CAD build for the part. Positions are in the model's coordinates, mm. A direction names the side the tool comes from. Coordinates: 2 decimals unless noted, no trailing zeros. Write item = value, one per line.
Autodesk Inventor part; units mm, degrees
ref_plane "C1_XY" through (0, 0, 0) normal (0, 0, 1) x (1, 0, 0)
ref_plane "C1_YZ" through (0, 0, 0) normal (1, 0, 0) x (0, 1, 0)
ref_plane "C1_ZX" through (0, 0, 0) normal (0, 1, 0) x (0, 0, 1)
sketch "Sketch_63" plane through (0, 0, 0) normal (0, 0, 1) x (1, 0, 0)
  line L0 (-10, -7) -> (-8, -7)
  line L1 (-8, -7) -> (-8, -4)
  line L2 (-8, -4) -> (-7.0607, -4)
  line L3 (-7.0607, -4) -> (-4, -7.0607)
  line L4 (-4, -7.0607) -> (-4, -9.4804)
  line L5 (-4, -9.4804) -> (-3.7, -10)
  line L6 (-3.7, -10) -> (-4, -10.5196)
  line L7 (-4, -10.5196) -> (-4, -12.9393)
  line L8 (-4, -12.9393) -> (-7.0607, -16)
  line L9 (-7.0607, -16) -> (-8, -16)
  line L10 (-8, -16) -> (-8, -13)
  line L11 (-8, -13) -> (-10, -13)
  line L12 (-10, -13) -> (-10, -19)
  arc A0 (-10, -19) -> (-9, -20) centre (-9, -19) ccw
  line L13 (-9, -20) -> (-3, -20)
  line L14 (-3, -20) -> (-3, -18)
  line L15 (-3, -18) -> (-6, -18)
  line L16 (-6, -18) -> (-6, -17.0607)
  line L17 (-6, -17.0607) -> (-2.9393, -14)
  line L18 (-2.9393, -14) -> (-0.5196, -14)
  line L19 (-0.5196, -14) -> (0, -13.7)
  line L20 (0, -13.7) -> (0.5196, -14)
  line L21 (0.5196, -14) -> (2.9393, -14)
  line L22 (2.9393, -14) -> (6, -17.0607)
  line L23 (6, -17.0607) -> (6, -18)
  line L24 (6, -18) -> (3, -18)
  line L25 (3, -18) -> (3, -20)
  line L26 (3, -20) -> (9, -20)
  arc A1 (9, -20) -> (10, -19) centre (9, -19) ccw
  line L27 (10, -19) -> (10, 19)
  arc A2 (10, 19) -> (9, 20) centre (9, 19) ccw
  line L28 (9, 20) -> (3, 20)
  line L29 (3, 20) -> (3, 18)
  line L30 (3, 18) -> (6, 18)
  line L31 (6, 18) -> (6, 17.0607)
  line L32 (6, 17.0607) -> (2.9393, 14)
  line L33 (2.9393, 14) -> (0.5196, 14)
  line L34 (0.5196, 14) -> (0, 13.7)
  line L35 (0, 13.7) -> (-0.5196, 14)
  line L36 (-0.5196, 14) -> (-2.9393, 14)
  line L37 (-2.9393, 14) -> (-6, 17.0607)
  line L38 (-6, 17.0607) -> (-6, 18)
  line L39 (-6, 18) -> (-3, 18)
  line L40 (-3, 18) -> (-3, 20)
  line L41 (-3, 20) -> (-9, 20)
  arc A3 (-9, 20) -> (-10, 19) centre (-9, 19) ccw
  line L42 (-10, 19) -> (-10, 13)
  line L43 (-10, 13) -> (-8, 13)
  line L44 (-8, 13) -> (-8, 16)
  line L45 (-8, 16) -> (-7.0607, 16)
  line L46 (-7.0607, 16) -> (-4, 12.9393)
  line L47 (-4, 12.9393) -> (-4, 10.5196)
  line L48 (-4, 10.5196) -> (-3.7, 10)
  line L49 (-3.7, 10) -> (-4, 9.4804)
  line L50 (-4, 9.4804) -> (-4, 7.0607)
  line L51 (-4, 7.0607) -> (-7.0607, 4)
  line L52 (-7.0607, 4) -> (-8, 4)
  line L53 (-8, 4) -> (-8, 7)
  line L54 (-8, 7) -> (-10, 7)
  line L55 (-10, 7) -> (-10, -7)
  line L56 (4, 12.9393) -> (4, 8.5)
  arc A4 (4, 8.5) -> (5, 7.5) centre (5, 8.5) ccw
  line L57 (5, 7.5) -> (7, 7.5)
  arc A5 (7, 7.5) -> (8, 8.5) centre (7, 8.5) ccw
  line L58 (8, 8.5) -> (8, 16)
  line L59 (8, 16) -> (7.0607, 16)
  line L60 (7.0607, 16) -> (4, 12.9393)
  line L61 (4, -12.9393) -> (7.0607, -16)
  line L62 (7.0607, -16) -> (8, -16)
  line L63 (8, -16) -> (8, -8.5)
  arc A6 (8, -8.5) -> (7, -7.5) centre (7, -8.5) ccw
  line L64 (7, -7.5) -> (5, -7.5)
  arc A7 (5, -7.5) -> (4, -8.5) centre (5, -8.5) ccw
  line L65 (4, -8.5) -> (4, -12.9393)
  line L66 (-8, 1.7) -> (-8, -1.7)
  arc A8 (-8, -1.7) -> (-7.7, -2) centre (-7.7, -1.7) ccw
  line L67 (-7.7, -2) -> (-7.0636, -2)
  arc A9 (-6.8515, -2.0879) -> (-7.0636, -2) centre (-7.0636, -2.3) ccw
  line L68 (-6.8515, -2.0879) -> (-2.9393, -6)
  line L69 (-2.9393, -6) -> (7, -6)
  arc A10 (7, -6) -> (8, -5) centre (7, -5) ccw
  line L70 (8, -5) -> (8, 5)
  arc A11 (8, 5) -> (7, 6) centre (7, 5) ccw
  line L71 (7, 6) -> (-2.9393, 6)
  line L72 (-2.9393, 6) -> (-6.8515, 2.0879)
  arc A12 (-7.0636, 2) -> (-6.8515, 2.0879) centre (-7.0636, 2.3) ccw
  line L73 (-7.0636, 2) -> (-7.7, 2)
  arc A13 (-7.7, 2) -> (-8, 1.7) centre (-7.7, 1.7) ccw
extrude "Extrusion1" add sketch "Sketch_63" against normal blind 393
sketch "Sketch2" plane through (0, 0, -393) normal (0, 0, -1) x (-1, 0, 0)
  point P0 (0, 10)
hole "Hole1" at (0, 10, -393) direction (0, 0, 1) diameter 4.2 end through all
pattern_linear "Rectangular Pattern1" count 2 spacing 20 along (0, -1, 0) of "Hole1"
ref_plane "C1_XY" through (0, 0, 0) normal (0, 0, 1) x (1, 0, 0)
ref_plane "C1_YZ" through (0, 0, 0) normal (1, 0, 0) x (0, 1, 0)
ref_plane "C1_ZX" through (0, 0, 0) normal (0, 1, 0) x (0, 0, 1)
thread "Thread1"
thread "Thread2"
thread "Thread3"
thread "Thread4"
properties part number "HFSF5-2040-393" material "Aluminum 6061"
(1) Wall check: line 1 (X direction, y = 10, z = -259); line 2 (Y direction, x = 0, z = -243); line 3 (Y direction, x = -9, z = -76). Give the ranges that are in metal, low to high. Write a range as from..to.
Evaluation:
line_1 = -3.7..-2.1, 2.1..4, 8..10
line_2 = -13.7..-12.1, -7.9..-6, 6..7.9, 12.1..13.7
line_3 = -20..-13, -7..7, 13..20
(2) Pull direction X, two halves, no side cores. Call faces 1 (the face through (8, 0, -194)), 2 (the face through (-10, 16, -194)), 3 (the face through (-6, 20, -194)): +X half, -X half, draft (parallel to the pull), parting line (faces both ways), or undercut.
Evaluation:
face_1 = undercut
face_2 = -X half
face_3 = draft
(3) Pin check, flat tips, straight feed: pin 1 Ø1 at (x, z) = (-9.5, -251.5) entering from -Y; pin 2 Ø1.2 at (y, z) = (8, -103.5) entering from -X; pin 3 Ø3 at (x, z) = (0, -85.5) entering from +Y; pin 4 Ø2 at (x, z) = (-1, -106) entering from -Y. Stop position of each tip, or through.
Evaluation:
pin_1 = -20
pin_2 = -4
pin_3 = 14
pin_4 = -14
(4) Slice it at A-A, the plane z = -202. State how many separate pieces and enclosed holes the cut face has, then the cut area to 3 significant figures.
Evaluation:
separate_pieces = 1
enclosed_holes = 5
area = 343 mm²
(5) Tool access for faces 4 (the face through (-5, 5, 0)), 5 (the face through (2, 6, -194)): list every direction of +Z, -Z, +X, -X, +Y, -Y with a clear straight run to the whole face (end or side of a thin tool).
Evaluation:
face_4 = +Z, +X, -X, +Y, -Y
face_5 = +Z, -Z
